from build123d import *

# Parameters (mm, degrees)
F0_W     = 20
F0_H     = 40
F1_DEPTH = 5
F2_W     = 5
F2_H     = 2
F3_DEPTH = 40.001
F4_R     = 4.99999


# Not quite as in the source:
# - a fillet or chamfer is up to 0.001 mm smaller than in the source, because OpenCascade refuses the exact size


with BuildPart() as f1:
    # F0 (on Front) → F1 (new body)
    with BuildSketch(Plane.XZ):
        Rectangle(F0_W, F0_H)
    extrude(amount=F1_DEPTH)

    # F2 (on face) → F3 (cut, through all)
    with BuildSketch(Plane(origin=(0, 0, -20), x_dir=(1, 0, 0), z_dir=(0, 0, -1))):
        with Locations((-2.5, 4)):
            Rectangle(F2_W, F2_H)
        with Locations((2.5, 4)):
            Rectangle(F2_W, F2_H)
    extrude(amount=-F3_DEPTH, mode=Mode.SUBTRACT)

    # F4 (radius 5 in the source; OpenCascade refuses exactly that, so slightly less here)
    f4_edges = [f1.edges().sort_by_distance(p)[0] for p in [
        (-10, -2.5, -20),
        (10, -2.5, -20),
        (-10, -2.5, 20),
        (10, -2.5, 20),
    ]]
    fillet(f4_edges, radius=F4_R)


solid = f1.part
Work out the finished part from the listing and answer in its coordinate system (mm). A direction names the side the tool comes from. Round coordinates to 2 decimals unless told otherwise and drop trailing zeros. Write each loop counter-clockwise with the first axis right and the second up, starting at its lowest first coordinate (ties: lowest second). Pieces come first, ordered by that corner, then holes. Notation, with made-up numbers: M -24,-9.5 L -19,-9.5 A12 cw -19,13.5 Z; hole C 50.25,26 d8. An arc over 180 degrees is marked long. Use a Markdown table: item, result.
1) A flat-ended cylindrical pin translates along its axis: pin 1 (8 mm diameter, centred on x = -4.5, z = 8, fed in from +Y). Find the tip coordinate at first contact, or state that the pin passes through.
Taken from the geometry:
| item | result |
|---|---|
| pin 1 | stops at y = 0 |
2) The part is cut by section B-B on z = 12.5. Give the vertices of the cut face in (x, y).
Taken from the geometry:
| item | result |
|---|---|
| outline | M -10,-5 L -5,-5 L -5,-3 L 5,-3 L 5,-5 L 10,-5 L 10,0 L -10,0 Z |
3) The part is cut by section D-D on z = 17. Give the vertices of the cut face in (x, y), plus the area to 3 significant figures.
Taken from the geometry:
| item | result |
|---|---|
| outline | M -9.58,-5 L -5,-5 L -5,-3 L 5,-3 L 5,-5 L 9.58,-5 L 9.58,0 L -9.58,0 Z |
| area | 75.8 mm2 |
4) Which of the six approach directions +Z, -Z, +X, -X, +Y, -Y give full straight-line access (tool end or side, diameter ignored) to faces 1 (the face through (7, -5, 0)), 2 (the face through (0, -3, 0))?
Taken from the geometry:
| item | result |
|---|---|
| face 1 | +Z, -Z, +X, -X, -Y |
| face 2 | +Z, -Z, -Y |
5) Consider line 1 (X direction, y = -4.45, z = 10); line 2 (Y direction, x = 0, z = -3); line 3 (X direction, y = -4.4, z = -18). Determine where each line is inside the solid, lowest interval first. Write a range as [from, to].
Taken from the geometry:
| item | result |
|---|---|
| line 1 | x = [-10, -5], [5, 10] |
| line 2 | y = [-3, 0] |
| line 3 | x = [-9, -5], [5, 9] |
6) The part is cut by section C-C on x = -9. Give the vertices of the cut face in (y, z), plus the area to 3 significant figures.
Taken from the geometry:
| item | result |
|---|---|
| outline | M -5,-18 L 0,-18 L 0,18 L -5,18 Z |
| area | 180 mm2 |
7) Determine the mould class of faces 3 (the face through (-9, -3, -18)), 4 (the face through (5, -4, 0)), 5 (the face through (0, -1, -20)) for opening direction X: pulls with the +X half, pulls with the -X half, needs draft (parallel to the pull), parting line crosses it, or undercut.
Taken from the geometry:
| item | result |
|---|---|
| face 3 | pulls with the -X half |
| face 4 | undercut |
| face 5 | needs draft |
